Job drawing, mm, ordinate dimensions from the low corner. One solid piece. A direction names the side the tool comes from. Coordinates: 2 decimals unless noted, no trailing zeros. Write each loop counter-clockwise with the first axis right and the second up, starting at its lowest first coordinate (ties: lowest second). Pieces come first, ordered by that corner, then holes. Notation, with made-up numbers: (44.5, -9) -> (58.5, -9) arc R31 cw to (58.5, 22) -> close; hole circle Ø4 at (50.25, 71). An arc over 180 degrees is marked (long way). One line per question, with ' | ' between items. Start each with the question number.
Item 1: Two-plate mould, pull along X, no slides. Class the marked faces 1, 2 and 3: pulls with the +X half, pulls with the -X half, needs draft (parallel to the pull), parting line crosses it, or undercut.
Item 2: Pin check, flat tip, straight feed: pin 1 (3 mm diameter, centred on x = 4.6, y = 4.6, fed in from -Z). Stop position of the tip, or through.
Item 3: 3-axis set-ups, long thin cutter, end or side, ignore diameter. For the marked faces 4 and 5: which of +Z, -Z, +X, -X, +Y, -Y reach the whole face in a straight line?
Item 4: Saw through at B-B (z = 2.85). List the corners of the cut face in (x, y), and give its area (3 significant figures).
Item 5: Saw through at C-C (z = 0.85). List the corners of the cut face in (x, y), and give its area (3 significant figures).
Item 6: Probe probe 1 along Y at (x, z) = (4.6, 0.95); probe 2 along Y at (x, z) = (4.6, 2.3); probe 3 along X at (y, z) = (5.5, 2.9). List the from-to ranges inside material, lowest first. Write a range as [from, to].
Item 7: Saw through at A-A (x = 4.6). List the corners of the cut face in (y, z), and give its area (3 significant figures).
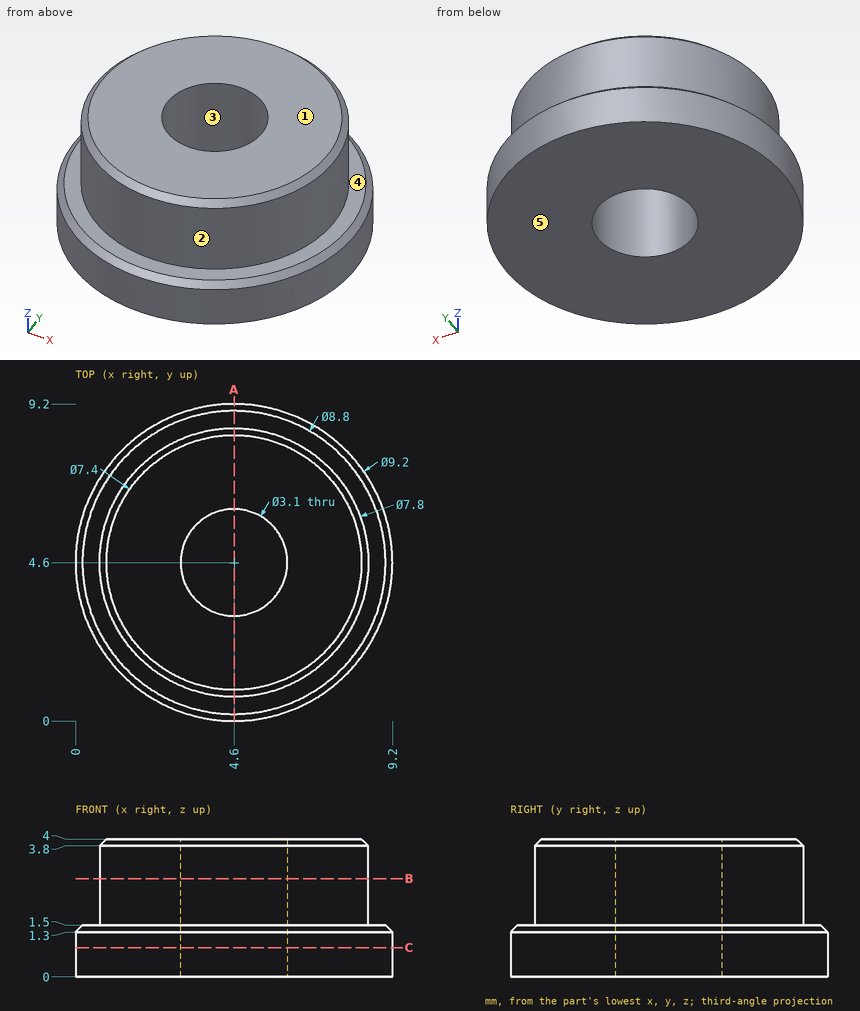
From the geometry:
1) face 1: needs draft | face 2: parting line crosses it | face 3: undercut
2) pin 1: through
3) face 4: +Z | face 5: -Z, +X, -X, +Y, -Y
4) outline: circle Ø7.8 at (4.6, 4.6); hole circle Ø3.1 at (4.6, 4.6) | area: 40.2 mm2
5) outline: circle Ø9.2 at (4.6, 4.6); hole circle Ø3.1 at (4.6, 4.6) | area: 58.9 mm2
6) probe 1: [0, 3.05], [6.15, 9.2] | probe 2: [0.7, 3.05], [6.15, 8.5] | probe 3: [0.81, 3.34], [5.86, 8.39]
7) outline: (0, 0) -> (3.05, 0) -> (3.05, 4) -> (0.9, 4) -> (0.7, 3.8) -> (0.7, 1.5) -> (0.2, 1.5) -> (0, 1.3) -> close; (6.15, 0) -> (9.2, 0) -> (9.2, 1.3) -> (9, 1.5) -> (8.5, 1.5) -> (8.5, 3.8) -> (8.3, 4) -> (6.15, 4) -> close | area: 20.8 mm2
